Here's the drawing with two shaded views (mm, measured from the low corner). I have some questions. Round coordinates to 2 decimals unless told otherwise and drop trailing zeros. Write each loop counter-clockwise with the first axis right and the second up, starting at its lowest first coordinate (ties: lowest second). Pieces come first, ordered by that corner, then holes. Notation, with made-up numbers: M 76,12.5 L 120,12.5 A28 ccw 120,38.5 Z; hole C 89,14 d2. An arc over 180 degrees is marked long. Answer as a JSON object with one key per item and string values. Group by question number.
1) Suppose I cut it at A-A, the plane x = 40. Write out the boundary of the cut face in (y, z), and give its area (3 significant figures).
2) Suppose I cut it at D-D, the plane x = 70. Write out the boundary of the cut face in (y, z), and give its area (3 significant figures).
3) Suppose I cut it at B-B, the plane y = 16. Write out the boundary of the cut face in (x, z), and give its area (3 significant figures).
4) I'm going to push flat-ended pins straight in: pin 1 Ø6 at (x, z) = (89, 8.5) entering from -Y; pin 2 Ø4 at (x, z) = (40, 9) entering from +Y. Where does each tip first touch, or does it pass through?
5) Please list where these lines run through material, in increasing order: L1, parallel to Z at x = 40, y = 14.25; L2, parallel to X at y = 22.25, z = 6.75; L3, parallel to X at y = 18.5, z = 10.5. Write a range as [from, to].
6) If we mould it in two halves opening along X, with no side actions, what happens to the marked faces 1, 2, 3 and 4? For each: +X half, -X half, draft (parallel to the pull), parting line (faces both ways), or undercut.
7) Suppose I cut it at C-C, the plane z = 4. Write out the boundary of the cut face in (x, y).
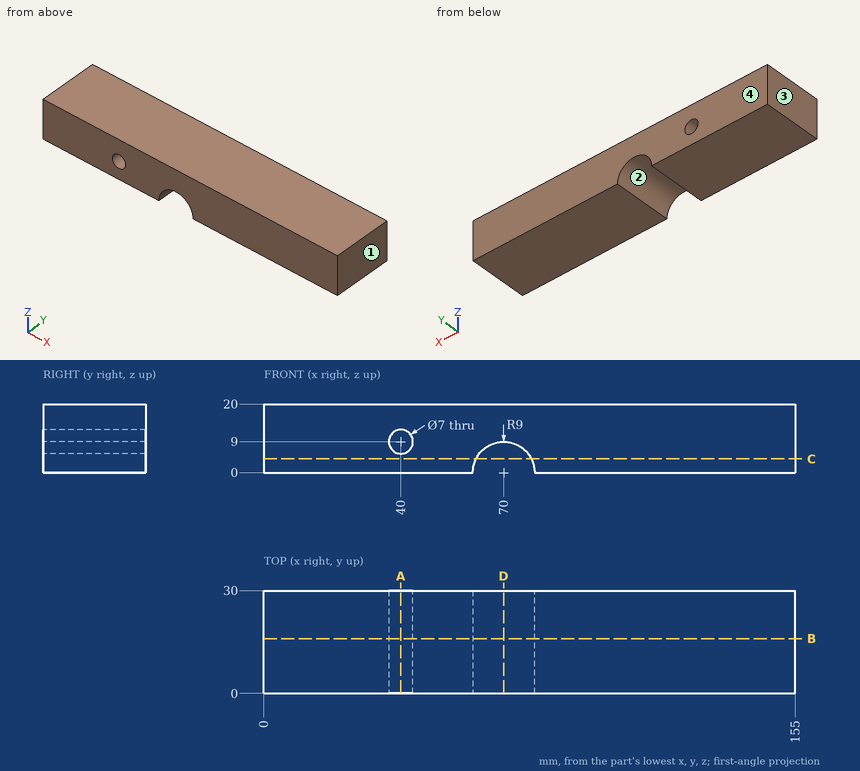
Results:
{
 "1": {"outline": "M 0,0 L 30,0 L 30,5.5 L 0,5.5 Z; M 0,12.5 L 30,12.5 L 30,20 L 0,20 Z", "area": "390 mm^2"},
 "2": {"outline": "M 0,9 L 30,9 L 30,20 L 0,20 Z", "area": "330 mm^2"},
 "3": {"outline": "M 0,0 L 61,0 A9 cw 79,0 L 155,0 L 155,20 L 0,20 Z; hole C 40,9 d7", "area": "2,930 mm^2"},
 "4": {"pin 1": "y = 0", "pin 2": "through"},
 "5": {"L1": "[0, 5.5], [12.5, 20]", "L2": "[0, 37.32], [42.68, 64.05], [75.95, 155]", "L3": "[0, 36.84], [43.16, 155]"},
 "6": {"face 1": "+X half", "face 2": "undercut", "face 3": "-X half", "face 4": "draft"},
 "7": {"outline": "M 0,0 L 61.94,0 L 61.94,30 L 0,30 Z; M 78.06,0 L 155,0 L 155,30 L 78.06,30 Z"}
}
